Geometry: final body of the model. Coordinates: model frame, mm. Face numbers are marked on the shaded views. Round coordinates to 2 decimals unless told otherwise and drop trailing zeros. Loops run counter-clockwise (first coordinate to the right, second up) from the corner with the lowest first, then second, coordinate; pieces in that order, holes last. Notation, with made-up numbers: (4, 34.5) - (57, 34.5) arc R36 cw to (57, 71.5) - close; hole circle Ø6 at (47, 33). An arc over 180 degrees is marked (long way). Return JSON: item names as keys, results as strings. Group by question number.
1. First-contact query: pin 1 Ø0.5 at (y, z) = (-9.5, 2.5) entering from -X; pin 2 Ø1.1 at (y, z) = (-9.5, 7) entering from +X; pin 3 Ø1.1 at (x, z) = (0.5, 4.5) entering from -Y. Flat tips, straight axial feed; report the tip coordinate or a pass-through.
2. Section D-D on x = 2. Return loops of the section in (y, z), and give its area (3 significant figures).
3. Material intervals for probe 1 along Z at (x, y) = (0.5, -5.5); probe 2 along Z at (x, y) = (5.25, -9.5); probe 3 along X at (y, z) = (-7.5, 6.25), sorted ascending.
4. Section B-B on x = 10. Return loops of the section in (y, z).
5. Section C-C on z = 4.5. Return loops of the section in (x, y).
6. Section A-A on y = -7.5. Return loops of the section in (x, z), and give its area (3 significant figures).
7. Draft query along Z for the marked faces 1, 2 and 3. Return one class per face: +Z half, -Z half, draft (parallel to the pull), parting line (faces both ways), or undercut.
from build123d import *

# Parameters (mm, degrees)
SKETCH1_W           = 22
SKETCH1_H           = 10
BOSS_EXTRUDE1_DEPTH = 9
FILLET2_R           = 0.5
CUT_EXTRUDE4_DEPTH  = 1
SKETCH8_W           = 2
SKETCH8_H           = 6.5
CUT_EXTRUDE5_DEPTH  = 1
CUT_EXTRUDE6_DEPTH  = 1
SKETCH13_R          = 0.45
FILLET3_R           = 0.1


with BuildPart() as part:
    # Sketch1 → Boss-Extrude1 (new body)
    with BuildSketch(Plane.XY):
        with Locations((11, -5)):
            Rectangle(SKETCH1_W, SKETCH1_H)
    extrude(amount=BOSS_EXTRUDE1_DEPTH)

    # Fillet2
    fillet2_edges = [part.edges().sort_by_distance(p)[0] for p in [
        (11, 0, 9),
        (11, 0, 0),
        (11, -10, 0),
        (11, -10, 9),
    ]]
    fillet(fillet2_edges, radius=FILLET2_R)

    # 3DSketch1 → Cut-Extrude4 (cut)
    with BuildSketch(Plane(origin=(22, -10, 5.5), x_dir=(0, 0.9557790087219501, -0.29408584883752314), z_dir=(1, 0, 0))):
        Polygon((0, 0), (6.212563557, 1.911558017), (6.800735254, 0), (0.588171698, -1.911558017), align=None)
    extrude(amount=-CUT_EXTRUDE4_DEPTH, mode=Mode.SUBTRACT)

    # Sketch8 → Cut-Extrude5 (cut)
    with BuildSketch(Plane.ZY):
        with Locations((4.5, -6.75)):
            Rectangle(SKETCH8_W, SKETCH8_H)
    extrude(amount=-CUT_EXTRUDE5_DEPTH, mode=Mode.SUBTRACT)

    # Sketch6 → Cut-Extrude6 (cut)
    with BuildSketch(Plane.XZ.offset(10)):
        Polygon((1, 5.5), (1, 3.5), (3, 3.5), (3, 1), (19, 1), (19, 3.5), (21, 3.5), (21, 5.5), (19, 5.5), (19, 8), (3, 8), (3, 5.5), align=None)
    extrude(amount=-CUT_EXTRUDE6_DEPTH, mode=Mode.SUBTRACT)

    # Sweep1: sweep along a curve in space
    with BuildLine() as sweep1_path:
        Line((21, -5, 4.5), (23.5, -5, 4.5))
        ThreePointArc((24.5, -6, 4.5), (24.207106781, -5.292893219, 4.5), (23.5, -5, 4.5))
        Line((24.5, -6, 4.5), (24.5, -13, 4.5))
    # Sketch13 → Sweep1 (sweep)
    with BuildSketch(Plane(origin=(21, 0, 0), x_dir=(0, 0, -1), z_dir=(1, 0, 0))):
        with Locations((-4.5, -5)):
            Circle(SKETCH13_R)
    sweep1 = sweep(path=sweep1_path.line)

    # Mirror1: Sweep1 across plane
    add(sweep1.mirror(Plane(origin=(11, 0, 0), x_dir=(0, 0, 1), z_dir=(1, 0, 0))))

    # Fillet3
    fillet3_edges = [part.edges().sort_by_distance(p)[0] for p in [
        (24.5, -13, 4.95),
        (-2.5, -13, 4.95),
    ]]
    fillet(fillet3_edges, radius=FILLET3_R)


solid = part.part
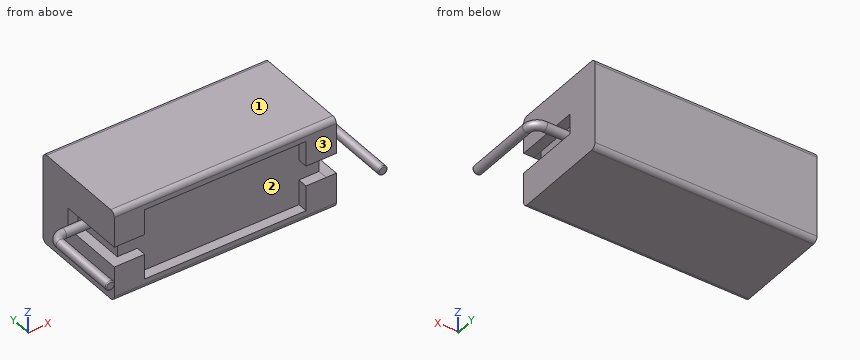
Taken from the geometry:
{
 "1": {"pin 1": "x = 0", "pin 2": "x = 22", "pin 3": "y = -9"},
 "2": {"outline": "(-10, 0.5) arc R0.5 ccw to (-9.5, 0) - (-0.5, 0) arc R0.5 ccw to (0, 0.5) - (0, 8.5) arc R0.5 ccw to (-0.5, 9) - (-9.5, 9) arc R0.5 ccw to (-10, 8.5) - (-10, 5.5) - (-9, 5.5) - (-9, 3.5) - (-10, 3.5) - close", "area": "87.8 mm2"},
 "3": {"probe 1": "0 to 3.5, 5.5 to 9", "probe 2": "0 to 1, 8 to 9", "probe 3": "0 to 22"},
 "4": {"outline": "(-10, 0.5) arc R0.5 ccw to (-9.5, 0) - (-0.5, 0) arc R0.5 ccw to (0, 0.5) - (0, 8.5) arc R0.5 ccw to (-0.5, 9) - (-9.5, 9) arc R0.5 ccw to (-10, 8.5) - (-10, 8) - (-9, 8) - (-9, 1) - (-10, 1) - close"},
 "5": {"outline": "(-2.95, -12.9) arc R0.1 ccw to (-2.85, -13) - (-2.15, -13) arc R0.1 ccw to (-2.05, -12.9) - (-2.05, -6) arc R0.55 cw to (-1.5, -5.45) - (1, -5.45) - (1, -9) - (21, -9) - (21, -5.45) - (23.5, -5.45) arc R0.55 cw to (24.05, -6) - (24.05, -12.9) arc R0.1 ccw to (24.15, -13) - (24.85, -13) arc R0.1 ccw to (24.95, -12.9) - (24.95, -6) arc R1.45 ccw to (23.5, -4.55) - (21, -4.55) - (21, -3.5) - (22, -3.5) - (22, 0) - (0, 0) - (0, -3.5) - (1, -3.5) - (1, -4.55) - (-1.5, -4.55) arc R1.45 ccw to (-2.95, -6) - close"},
 "6": {"outline": "circle Ø0.9 at (-2.5, 4.5); (0, 0) - (22, 0) - (22, 3.5) - (21, 3.5) - (21, 5.5) - (22, 5.5) - (22, 9) - (0, 9) - (0, 5.5) - (1, 5.5) - (1, 3.5) - (0, 3.5) - close; circle Ø0.9 at (24.5, 4.5)", "area": "195 mm2"},
 "7": {"face 1": "+Z half", "face 2": "undercut", "face 3": "draft"}
}
